Could you check a few things on this model? Use its own coordinates, in mm. Coordinates: 2 decimals unless noted, no trailing zeros. Loops run counter-clockwise (first coordinate to the right, second up) from the corner with the lowest first, then second, coordinate; pieces in that order, holes last. Notation, with made-up numbers: M 16.25,20 L 53.25,20 A26 cw 53.25,43 Z; hole C 68.5,22 d11. An arc over 180 degrees is marked long. Return JSON: item names as keys, results as strings. Group by question number.
from build123d import *

# Parameters (mm, degrees)
SKETCH1_R                      = 1
BOSS_EXTRUDE1_DEPTH            = 2
M3_CLEARANCE_HOLE1_D           = 3.6
M3_CLEARANCE_HOLE1_CSINK_D     = 3.65
M3_CLEARANCE_HOLE1_CSINK_ANGLE = 90


with BuildPart() as part:
    # Sketch1 → Boss-Extrude1 (new, symmetric)
    with BuildSketch(Plane(origin=(0, 0, 0), x_dir=(1, 0, 0), z_dir=(0, 1, 0))):
        with BuildLine():
            Line((0, 4), (120, 4))
            ThreePointArc((120, 4), (124, 0), (120, -4))
            Line((120, -4), (0, -4))
            ThreePointArc((0, -4), (-4, 0), (0, 4))
        make_face()
        with Locations(Location((0, 0, 0), (0, 0, 270))):
            Circle(SKETCH1_R, mode=Mode.SUBTRACT)
        with Locations(Location((120, 0, 0), (0, 0, 270))):
            Circle(SKETCH1_R, mode=Mode.SUBTRACT)
        with Locations(Location((110, 0, 0), (0, 0, 270))):
            Circle(SKETCH1_R, mode=Mode.SUBTRACT)
    extrude(amount=BOSS_EXTRUDE1_DEPTH, both=True)

    # Sketch3 → Cut-Revolve1 (revolve, cut)
    with BuildSketch(Plane.XY, mode=Mode.PRIVATE) as cut_revolve1_sk:
        with BuildLine():
            Line((110, 2), (112.163762696, 2))
            Line((112.163762696, 2), (111.560307379, 0.342020143))
            ThreePointArc((111.560307379, 0.342020143), (111.5, 0), (111.560307379, -0.342020143))
            Line((111.560307379, -0.342020143), (112.163762696, -2))
            Line((112.163762696, -2), (110, -2))
            Line((110, -2), (110, 2))
        make_face()
    revolve(cut_revolve1_sk.sketch.rotate(Axis((110, 2, 0), (0, -1, 0)), 90), axis=Axis((110, 2, 0), (0, -1, 0)), mode=Mode.SUBTRACT)

    # M3 Clearance Hole1 (through all)
    with Locations(Plane(origin=(0, 2, 0), x_dir=(1, 0, 0), z_dir=(0, 1, 0))):
        with Locations((0, 0), (120, 0)):
            CounterSinkHole(M3_CLEARANCE_HOLE1_D / 2, M3_CLEARANCE_HOLE1_CSINK_D / 2, counter_sink_angle=M3_CLEARANCE_HOLE1_CSINK_ANGLE)


solid = part.part
(1) Imagine slicing it at B-B, the plane z = 0. Write out the boundary of the cut face in (x, y) (3 decimals).
(2) Imagine slicing it at A-A, the plane x = 110. Write out the boundary of the cut face in (y, z), then the cut area to 3 significant figures.
(3) We'd pull the mould along Z, two halves only. Please class faces 1 (the face through (-4, 0, 0)), 2 (the face through (61, -2, 0)), 3 (the face through (-1.717, -0.04, -0.541)): +Z half, -Z half, draft (parallel to the pull), parting line (faces both ways), or undercut.
(4) Imagine slicing it at C-C, the plane y = 1.1. Write out the boundary of the cut face in (x, z).
(5) If I drill on L1, parallel to Z at x = 120, y = 0.4; L2, parallel to X at y = -0.55, z = -1.25; L3, parallel to X at y = 1.65, z = -0.5, over which ranges is the centre line in solid material (lowest first)? Write a range as [from, to].
(6) Will this pin go through, and if not, where does the flat tip stop? P1, Ø2, axis at y = 1.5, z = -2, coming from the -X side.
Checks:
{
 "1": {"outline": "M -4,-2 L -1.8,-2 L -1.8,1.975 L -1.825,2 L -4,2 Z; M 1.8,-2 L 107.836,-2 L 108.44,-0.342 A1 ccw 108.44,0.342 L 107.836,2 L 1.825,2 L 1.8,1.975 Z; M 111.56,-0.342 L 112.164,-2 L 118.2,-2 L 118.2,1.975 L 118.175,2 L 112.164,2 L 111.56,0.342 A1 ccw Z; M 121.8,-2 L 124,-2 L 124,2 L 121.825,2 L 121.8,1.975 Z"},
 "2": {"outline": "M -2,-4 L 2,-4 L 2,-2.16 L 0.34,-1.56 A1 ccw -0.34,-1.56 L -2,-2.16 Z; M -2,2.16 L -0.34,1.56 A1 ccw 0.34,1.56 L 2,2.16 L 2,4 L -2,4 Z", "area": "17.6 mm²"},
 "3": {"face 1": "parting line", "face 2": "draft", "face 3": "undercut"},
 "4": {"outline": "M 0,-4 L 120,-4 A4 ccw 120,4 L 0,4 A4 ccw Z; hole C 0,0 d3.6; hole C 110,0 d3.67; hole C 120,0 d3.6"},
 "5": {"L1": "[-4, -1.8], [1.8, 4]", "L2": "[-3.8, -1.3], [1.3, 108.94], [111.06, 118.7], [121.3, 123.8]", "L3": "[-3.97, -1.73], [1.73, 108.03], [111.97, 118.27], [121.73, 123.97]"},
 "6": {"P1": "x = -3.87"}
}
